For this review, take the finished solid that the model builds, in its own axes (mm). Face numbers are marked on the shaded views. A direction names the side the tool comes from. Coordinates: 2 decimals unless noted, no trailing zeros. Write each loop counter-clockwise with the first axis right and the second up, starting at its lowest first coordinate (ties: lowest second). Pieces come first, ordered by that corner, then holes. Notation, with made-up numbers: (-21.5, 5) -> (17.5, 5) arc R32 ccw to (17.5, 33) -> close; hole circle Ø10 at (28.25, 61). An arc over 180 degrees is marked (long way). Put each result on its own line as item: value. Start each with the question number.
Item 1: Consider section A-A on y = 0. Give the boundary of the cut face in (x, z).
Item 2: The part is to be moulded in two halves that separate along X. For the marked faces 1, 2 and 3, say which applies: +X half, -X half, draft (parallel to the pull), parting line (faces both ways), or undercut.
Item 3: Consider section C-C on x = 0. Give the boundary of the cut face in (y, z).
Item 4: For the marked faces 4 and 5, list the 3-axis set-ups (+Z, -Z, +X, -X, +Y, -Y) from which the entire face can be reached by the end or side of a thin tool; tool diameter is ignored.
Item 5: Insertion check: P1, Ø2.5, axis at x = 1, y = 0.5, coming from the -Z side; P2, Ø10, axis at x = -26, y = 7, coming from the +Z side; P3, Ø8, axis at x = 0, y = 0, coming from the -Z side; P4, Ø1.6, axis at y = 0.5, z = 140.5, coming from the -X side. Each pin has a flat end and moves straight along its axis. Give the tip position at first contact, or say it passes through.
Item 6: Consider section D-D on y = -16.5. Give the boundary of the cut face in (x, z).
Item 7: Consider section B-B on z = 112.5. Give the boundary of the cut face in (x, y).
Item 8: To check wall thickness, follow L1, parallel to X at y = 3.5, z = 125; L2, parallel to Y at x = 0, z = 2.1; L3, parallel to Z at x = -32.7, y = 0. State the ranges of each line that lie inside material, in increasing order.
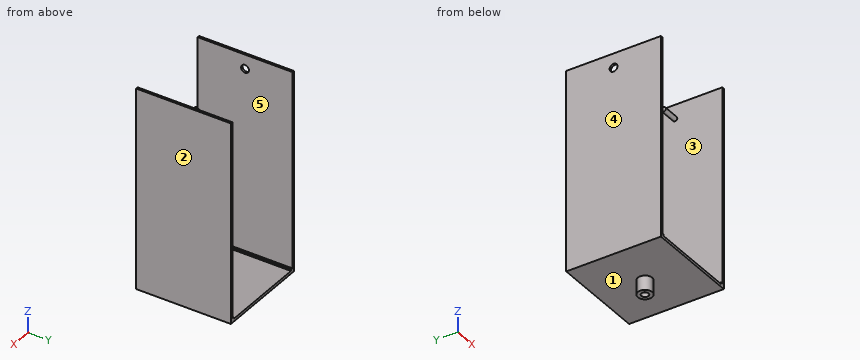
```python
from build123d import *

# Parameters (mm, degrees)
ESBO_O1_R                = 5
RESSALTO_EXTRUS_O2_DEPTH = 10
ESBO_O3_R                = 2.5
CORTE_EXTRUS_O2_DEPTH    = 3
ESBO_O4_W                = 66
ESBO_O4_H                = 66
RESSALTO_EXTRUS_O3_DEPTH = 60
ESBO_O5_W                = 60
ESBO_O5_H                = 63
CORTE_EXTRUS_O3_DEPTH    = 57
ESBO_O6_W                = 60
ESBO_O6_H                = 59
CORTE_EXTRUS_O5_DEPTH    = 84
ESBO_O7_W                = 2.941982117
ESBO_O7_H                = 66
ESBO_O7_W_2              = 3.058017883
RESSALTO_EXTRUS_O4_DEPTH = 80
ESBO_O8_W                = 1.470991058
ESBO_O8_H                = 66
ESBO_O8_W_2              = 1.529008942
CORTE_EXTRUS_O6_DEPTH    = 137
ESBO_O9_R                = 2.75
CORTE_EXTRUS_O7_DEPTH    = 49
ESBO_O10_R               = 1.6
RESSALTO_EXTRUS_O5_DEPTH = 12


with BuildPart() as part:
    # Esboço1 → Ressalto-extrusão2 (new body)
    with BuildSketch(Plane.XY):
        Circle(ESBO_O1_R)
    extrude(amount=RESSALTO_EXTRUS_O2_DEPTH)

    # Esboço3 → Corte-extrusão2 (cut)
    with BuildSketch(Plane(origin=(0, 0, 0), x_dir=(-1, 0, 0), z_dir=(0, 0, -1))):
        Circle(ESBO_O3_R)
    extrude(amount=-CORTE_EXTRUS_O2_DEPTH, mode=Mode.SUBTRACT)

    # Esboço4 → Ressalto-extrusão3 (add)
    with BuildSketch(Plane.XY.offset(10)):
        Rectangle(ESBO_O4_W, ESBO_O4_H)
    extrude(amount=RESSALTO_EXTRUS_O3_DEPTH)

    # Esboço5 → Corte-extrusão3 (cut)
    with BuildSketch(Plane.XY.offset(70)):
        Rectangle(ESBO_O5_W, ESBO_O5_H)
    extrude(amount=-CORTE_EXTRUS_O3_DEPTH, mode=Mode.SUBTRACT)

    # Esboço6 → Corte-extrusão5 (cut)
    with BuildSketch(Plane(origin=(0, 33, 0), x_dir=(1, 0, 0), z_dir=(0, 1, 0))):
        with Locations((-0.058017883, -41.456168944)):
            Rectangle(ESBO_O6_W, ESBO_O6_H)
    extrude(amount=-CORTE_EXTRUS_O5_DEPTH, mode=Mode.SUBTRACT)

    # Esboço7 → Ressalto-extrusão4 (add)
    with BuildSketch(Plane.XY.offset(70)):
        with Locations((-31.529008942, 0)):
            Rectangle(ESBO_O7_W, ESBO_O7_H)
        with Locations((31.470991059, 0)):
            Rectangle(ESBO_O7_W_2, ESBO_O7_H)
    extrude(amount=RESSALTO_EXTRUS_O4_DEPTH)

    # Esboço8 → Corte-extrusão6 (cut)
    with BuildSketch(Plane.XY.offset(150)):
        with Locations((-30.793513412, 0)):
            Rectangle(ESBO_O8_W, ESBO_O8_H)
        with Locations((30.706486588, 0)):
            Rectangle(ESBO_O8_W_2, ESBO_O8_H)
    extrude(amount=-CORTE_EXTRUS_O6_DEPTH, mode=Mode.SUBTRACT)

    # Esboço9 → Corte-extrusão7 (cut)
    with BuildSketch(Plane.ZY.offset(33)):
        with Locations(Location((140.048047336, 0, 0), (0, 0, 270))):
            Circle(ESBO_O9_R)
    extrude(amount=-CORTE_EXTRUS_O7_DEPTH, mode=Mode.SUBTRACT)

    # Esboço10 → Ressalto-extrusão5 (add)
    with BuildSketch(Plane.ZY.offset(-31.470991059)):
        with Locations(Location((140.048047336, 0, 0), (0, 0, 180))):
            Circle(ESBO_O10_R)
    extrude(amount=RESSALTO_EXTRUS_O5_DEPTH)


solid = part.part
```
Return value:
1. outline: (-33, 10) -> (-5, 10) -> (-5, 0) -> (-2.5, 0) -> (-2.5, 3) -> (2.5, 3) -> (2.5, 0) -> (5, 0) -> (5, 10) -> (33, 10) -> (33, 150) -> (31.47, 150) -> (31.47, 141.65) -> (19.47, 141.65) -> (19.47, 138.45) -> (31.47, 138.45) -> (31.47, 13) -> (29.94, 13) -> (29.94, 11.96) -> (-30.06, 11.96) -> (-30.06, 13) -> (-31.53, 13) -> (-31.53, 137.3) -> (-33, 137.3) -> close; (-33, 142.8) -> (-31.53, 142.8) -> (-31.53, 150) -> (-33, 150) -> close
2. face 1: draft
2. face 2: +X half
2. face 3: undercut
3. outline: (-33, 10) -> (-5, 10) -> (-5, 0) -> (-2.5, 0) -> (-2.5, 3) -> (2.5, 3) -> (2.5, 0) -> (5, 0) -> (5, 10) -> (33, 10) -> (33, 11.96) -> (-33, 11.96) -> close
4. face 4: +Z, -Z, -X, +Y, -Y
4. face 5: +Z, +Y, -Y
5. P1: z = 3
5. P2: z = 13
5. P3: z = 0
5. P4: x = 19.47
6. outline: (-33, 10) -> (33, 10) -> (33, 150) -> (31.47, 150) -> (31.47, 13) -> (29.94, 13) -> (29.94, 11.96) -> (-30.06, 11.96) -> (-30.06, 13) -> (-31.53, 13) -> (-31.53, 150) -> (-33, 150) -> close
7. outline: (-33, -33) -> (-31.53, -33) -> (-31.53, 33) -> (-33, 33) -> close; (31.47, -33) -> (33, -33) -> (33, 33) -> (31.47, 33) -> close
8. L1: -33 to -31.53, 31.47 to 33
8. L2: -5 to -2.5, 2.5 to 5
8. L3: 10 to 137.3, 142.8 to 150
